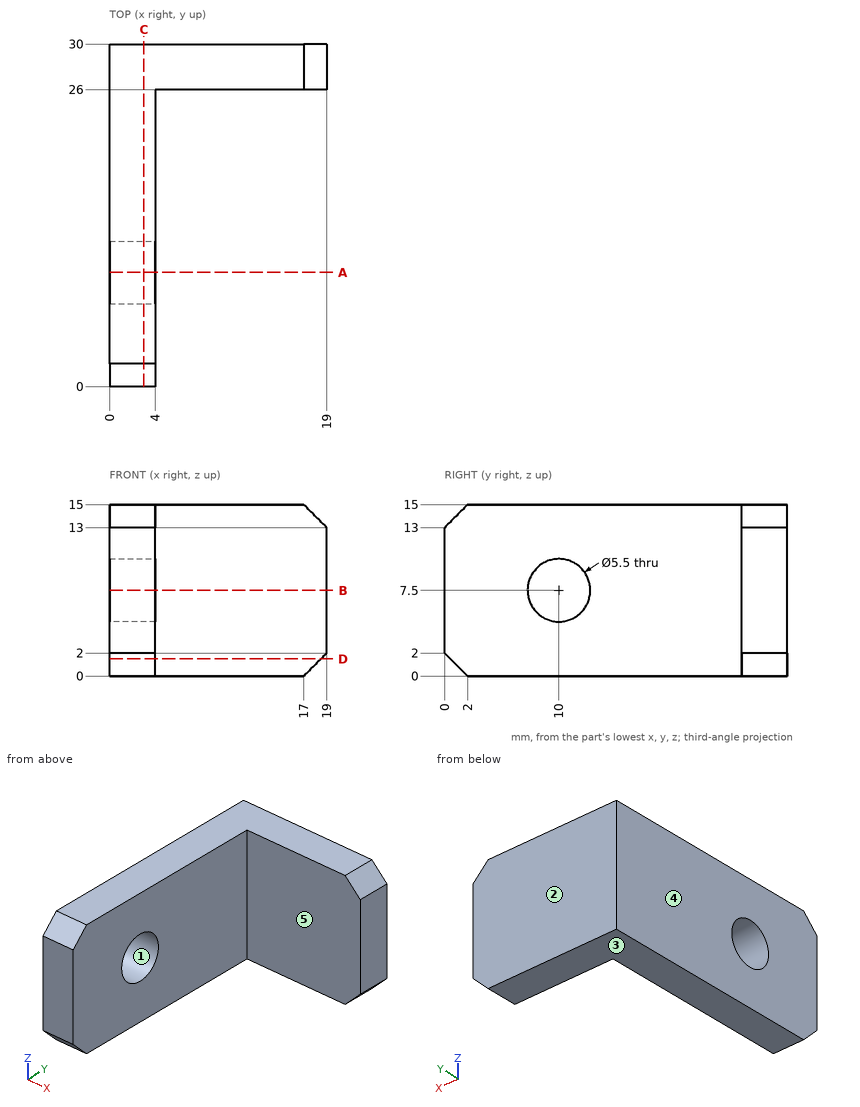
Study the drawing (mm; zero at the part's minimum x, y, z) and answer. A direction names the side the tool comes from. Give positions to 0.01 mm unless a question says otherwise; leave off trailing zeros. Write each loop counter-clockwise with the first axis right and the second up, starting at its lowest first coordinate (ties: lowest second). Pieces come first, ordered by that corner, then holes. Notation, with made-up numbers: (30, 83.25) -> (81, 83.25) arc R30 ccw to (81, 109.25) -> close; hole circle Ø3 at (-9.5, 9.5). An arc over 180 degrees is marked (long way). Answer as a JSON object with one key per item and string values. Group by question number.
1) Find section B-B (z = 7.5). Write down the section's boundary in (x, y), and give its area (3 significant figures).
2) Consider L1, parallel to Y at x = 2.75, z = 7.5; L2, parallel to X at y = 16, z = 9.25; L3, parallel to Y at x = 12.25, z = 6.5. Determine where each line is inside the solid, lowest interval first. Write a range as from..to.
3) Find section D-D (z = 1.5). Write down the section's boundary in (x, y), and give its area (3 significant figures).
4) Find section A-A (y = 10). Write down the section's boundary in (x, z), and give its area (3 significant figures).
5) A tool of negligible diameter and unlimited length cuts with its end or side. For the marked faces 4 and 5, from which of +Z, -Z, +X, -X, +Y, -Y can it reach the whole face along a straight path? Write none if from no direction.
6) Each of these flat-tipped pins is pushed along its axis until it touches: P1, Ø2, axis at x = 6, y = 21.5, coming from the +Z side; P2, Ø7.5, axis at y = 10.5, z = 5.5, coming from the +X side. Where does it stop, or does it pass through?
7) Find section C-C (x = 3). Write down the section's boundary in (y, z), and give its area (3 significant figures).
8) The mould has two halves that part along Y. Classify the marked faces 1, 2 and 3: +Y half, -Y half, draft (parallel to the pull), parting line (faces both ways), or undercut.
Values follow:
{
 "1": {"outline": "(0, 0) -> (4, 0) -> (4, 7.25) -> (0, 7.25) -> close; (0, 12.75) -> (4, 12.75) -> (4, 26) -> (19, 26) -> (19, 30) -> (0, 30) -> close", "area": "158 mm2"},
 "2": {"L1": "y = 0..7.25, 12.75..30", "L2": "x = 0..4", "L3": "y = 26..30"},
 "3": {"outline": "(0, 0.5) -> (4, 0.5) -> (4, 26) -> (18.5, 26) -> (18.5, 30) -> (0, 30) -> close", "area": "176 mm2"},
 "4": {"outline": "(0, 0) -> (4, 0) -> (4, 4.75) -> (0, 4.75) -> close; (0, 10.25) -> (4, 10.25) -> (4, 15) -> (0, 15) -> close", "area": "38.0 mm2"},
 "5": {"face 4": "+Z, -Z, -X, +Y, -Y", "face 5": "+Z, -Z, +X, -Y"},
 "6": {"P1": "passes through", "P2": "stops at x = 4"},
 "7": {"outline": "(0, 2) -> (2, 0) -> (30, 0) -> (30, 15) -> (2, 15) -> (0, 13) -> close; hole circle Ø5.5 at (10, 7.5)", "area": "422 mm2"},
 "8": {"face 1": "undercut", "face 2": "+Y half", "face 3": "draft"}
}
